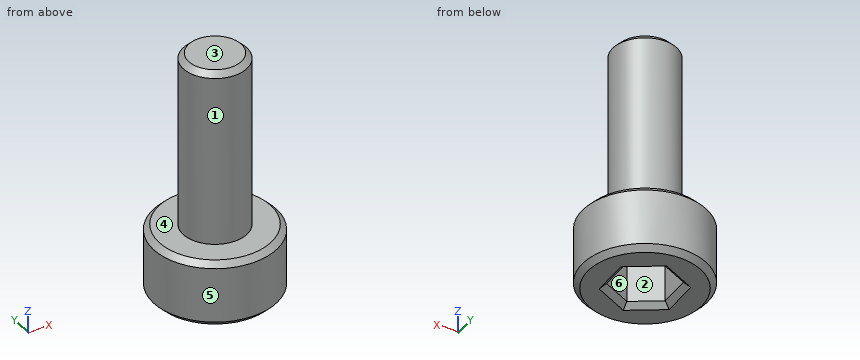
```python
from build123d import *

# Parameters (mm, degrees)
SKETCH_R     = 2.8
PAD_DEPTH    = 3
SKETCH001_R  = 1.45
PAD001_DEPTH = 8
POCKET_DEPTH = 2
CHAMFER_SIZE = 0.25


with BuildPart() as part:
    # Sketch → Pad (new body)
    with BuildSketch(Plane.XY):
        Circle(SKETCH_R)
    extrude(amount=PAD_DEPTH)

    # Sketch001 (on Face3 of Pad) → Pad001 (join)
    with BuildSketch(Plane.XY.offset(3)):
        Circle(SKETCH001_R)
    extrude(amount=PAD001_DEPTH)

    # Sketch002 (on Face2 of Pad001) → Pocket (cut)
    with BuildSketch(Plane(origin=(0, 0, 0), x_dir=(1, 0, 0), z_dir=(0, 0, -1))):
        Polygon((1.259542, 0.814588), (-0.075682, 1.49809), (-1.335225, 0.683502), (-1.259542, -0.814588), (0.075682, -1.49809), (1.335225, -0.683502), align=None)
    extrude(amount=-POCKET_DEPTH, mode=Mode.SUBTRACT)

    # Chamfer
    chamfer_edges = [part.edges().sort_by_distance(p)[0] for p in [
        (-2.8, 0, 3),
        (-2.8, 0, 0),
        (1.297384, -0.065543, 0),
        (0.705454, 1.090796, 0),
        (-0.59193, 1.156339, 0),
        (-1.297384, 0.065543, 0),
        (-0.705454, -1.090796, 0),
        (0.59193, -1.156339, 0),
        (-1.45, 0, 11),
    ]]
    chamfer(chamfer_edges, length=CHAMFER_SIZE)


solid = part.part
```
For this review, take the finished solid that the model builds, in its own axes (mm). Face numbers are marked on the shaded views. A direction names the side the tool comes from. Coordinates: 2 decimals unless noted, no trailing zeros. Order: outer loops, then holes, each group sorted by start corner. A loop starts at its lowest first (then second) coordinate and runs counter-clockwise, first axis right, second up. Notation, with made-up numbers: (23.25, 59) -> (53.25, 59) arc R24 cw to (53.25, 95) -> close; hole circle Ø2 at (0.25, 72.25). An arc over 180 degrees is marked (long way). Answer as CSV lines item,"result".
Q1. We need section B-B (z = 10). State the section outline as (x, y) points.
Model answer:
outline,"circle Ø2.9 at (0, 0)"
Q2. Wall thickness on line 1 along Z through (x, y) = (-0.05, 0.85); line 2 along Z through (x, y) = (0.65, 1.75); line 3 along X through (y, z) = (-0.75, 7.25): over which ranges is each line inside the solid? List them lowest first. Write a range as [from, to].
Model answer:
line 1,"z = [2, 11]"
line 2,"z = [0, 3]"
line 3,"x = [-1.24, 1.24]"
Q3. For the marked faces 1, 2 and 3, list the 3-axis set-ups (+Z, -Z, +X, -X, +Y, -Y) from which the entire face can be reached by the end or side of a thin tool; tool diameter is ignored.
Model answer:
face 1,"+Z"
face 2,"-Z"
face 3,"+Z, +X, -X, +Y, -Y"
Q4. We need section C-C (z = 2.5). State the section outline as (x, y) points, plus the area to 3 significant figures.
Model answer:
outline,"circle Ø5.6 at (0, 0)"
area,"24.6 mm2"
Q5. Clearance check with a flat-ended pin moving along its axis: pin 1 Ø1.5 at (x, z) = (0, 5.5) entering from -Y. State where the tip first meets the part, or that it passes through.
Model answer:
pin 1,"stops at y = -1.45"
Q6. We need section A-A (y = 0). State the section outline as (x, z) points.
Model answer:
outline,"(-2.8, 0.25) -> (-2.55, 0) -> (-1.55, 0) -> (-1.3, 0.25) -> (-1.3, 2) -> (1.3, 2) -> (1.3, 0.25) -> (1.55, 0) -> (2.55, 0) -> (2.8, 0.25) -> (2.8, 2.75) -> (2.55, 3) -> (1.45, 3) -> (1.45, 10.75) -> (1.2, 11) -> (-1.2, 11) -> (-1.45, 10.75) -> (-1.45, 3) -> (-2.55, 3) -> (-2.8, 2.75) -> close"
Q7. Draft analysis for pull direction X (two halves, no side actions). For the marked faces 4, 5 and 6, state which applies: released by +X, released by -X, zero draft, split by the parting line, or undercut.
Model answer:
face 4,"zero draft"
face 5,"split by the parting line"
face 6,"undercut"
